Build history of the part. All positions in model axes, mm. A direction names the side the tool comes from. Round coordinates to 2 decimals unless told otherwise and drop trailing zeros. Write each loop counter-clockwise with the first axis right and the second up, starting at its lowest first coordinate (ties: lowest second). Pieces come first, ordered by that corner, then holes.
from build123d import *

# Parameters (mm, degrees)
SKETCH1_W                                      = 127
SKETCH1_H                                      = 12.7
BOSS_EXTRUDE1_DEPTH                            = 38.1
SKETCH3_R                                      = 4.445
CUT_EXTRUDE3_DEPTH                             = 2.54
CUT_EXTRUDE4_DEPTH                             = 13.208
CUT_EXTRUDE4_DEPTH_BACK                        = 13.208
SKETCH2_R                                      = 7.9756
SKETCH2_R_2                                    = 8.1026
SKETCH6_R                                      = 5.08
CUT_EXTRUDE5_DEPTH                             = 38.1
F_11_64_0_17188_DIAMETER_HOLE1_D               = 4.365752
F_11_64_0_17188_DIAMETER_HOLE1_DEPTH           = 25.4
F_11_64_0_17188_DIAMETER_HOLE1_TIP             = 1.311604225
F_11_64_0_17188_DIAMETER_HOLE1_ON_FACE_2_D     = 4.365752
F_11_64_0_17188_DIAMETER_HOLE1_ON_FACE_2_DEPTH = 25.4
F_11_64_0_17188_DIAMETER_HOLE1_ON_FACE_2_TIP   = 1.311604225


with BuildPart() as part:
    # Sketch1 → Boss-Extrude1 (new body)
    with BuildSketch(Plane(origin=(0, 0, 0), x_dir=(1, 0, 0), z_dir=(0, 1, 0))):
        with Locations((0, -6.35)):
            Rectangle(SKETCH1_W, SKETCH1_H)
    extrude(amount=BOSS_EXTRUDE1_DEPTH)

    # Sketch3 → Cut-Extrude3 (cut)
    with BuildSketch(Plane(origin=(0, 0, 0), x_dir=(-1, 0, 0), z_dir=(0, 0, -1))):
        with Locations((-58.039, 31.75)):
            Circle(SKETCH3_R)
        with Locations((-58.039, 6.35)):
            Circle(SKETCH3_R)
        with Locations((-31.009232106, 31.75)):
            Circle(SKETCH3_R)
        with Locations((-31.009232106, 6.35)):
            Circle(SKETCH3_R)
        with Locations((31.009232106, 31.75)):
            Circle(SKETCH3_R)
        with Locations((31.009232106, 6.35)):
            Circle(SKETCH3_R)
        with Locations((58.039, 31.75)):
            Circle(SKETCH3_R)
        with Locations((58.039, 6.35)):
            Circle(SKETCH3_R)
    extrude(amount=-CUT_EXTRUDE3_DEPTH, mode=Mode.SUBTRACT)

    # Sketch2 → Cut-Extrude4 (cut, two sides: drawn at the far end of the back side and taken through both)
    with BuildSketch(Plane(origin=(0, 19.05, 0), x_dir=(1, 0, 0), z_dir=(0, 1, 0)).offset(-CUT_EXTRUDE4_DEPTH_BACK)):
        with Locations((-44.45, -13.97)):
            Circle(SKETCH2_R)
        with Locations((44.45, -13.97)):
            Circle(SKETCH2_R_2)
    extrude(amount=CUT_EXTRUDE4_DEPTH + CUT_EXTRUDE4_DEPTH_BACK, mode=Mode.SUBTRACT)

    # Sketch6 → Cut-Extrude5 (cut)
    with BuildSketch(Plane(origin=(0, 38.1, 0), x_dir=(1, 0, 0), z_dir=(0, 1, 0))):
        with Locations((-44.45, -13.97)):
            Circle(SKETCH6_R)
        with Locations((44.45, -13.97)):
            Circle(SKETCH6_R)
    extrude(amount=-CUT_EXTRUDE5_DEPTH, mode=Mode.SUBTRACT)

    # 11/64 (0.17188) Diameter Hole1
    with Locations(Plane(origin=(58.039, 31.75, 0), x_dir=(-1, 0, 0), z_dir=(0, 0, -1))):
        with Locations((0, 0), (27.029767894, 0), (27.029767894, -25.4), (89.048232106, -25.4), (116.078, 0)):
            Hole(F_11_64_0_17188_DIAMETER_HOLE1_D / 2, depth=F_11_64_0_17188_DIAMETER_HOLE1_DEPTH)
            with Locations((0, 0, -(F_11_64_0_17188_DIAMETER_HOLE1_DEPTH + F_11_64_0_17188_DIAMETER_HOLE1_TIP / 2))):  # 118° drill point
                Cone(0, F_11_64_0_17188_DIAMETER_HOLE1_D / 2, F_11_64_0_17188_DIAMETER_HOLE1_TIP, mode=Mode.SUBTRACT)

    # 11/64 (0.17188) Diameter Hole1 on face 2
    with Locations(Plane(origin=(58.039, 6.35, 2.54), x_dir=(-1, 0, 0), z_dir=(0, 0, -1))):
        with Locations((0, 0), (89.048232106, 25.4), (116.078, 0)):
            Hole(F_11_64_0_17188_DIAMETER_HOLE1_ON_FACE_2_D / 2, depth=F_11_64_0_17188_DIAMETER_HOLE1_ON_FACE_2_DEPTH)
            with Locations((0, 0, -(F_11_64_0_17188_DIAMETER_HOLE1_ON_FACE_2_DEPTH + F_11_64_0_17188_DIAMETER_HOLE1_ON_FACE_2_TIP / 2))):  # 118° drill point
                Cone(0, F_11_64_0_17188_DIAMETER_HOLE1_ON_FACE_2_D / 2, F_11_64_0_17188_DIAMETER_HOLE1_ON_FACE_2_TIP, mode=Mode.SUBTRACT)


solid = part.part
1) Slice it at A-A (z = 3.75). Count the separate pieces of the cut face and the enclosed holes in it, plus the area to 3 significant figures.
Results:
separate pieces: 1
enclosed holes: 8
area: 4,720 mm2
2) Wall check: L1, parallel to Y at x = -58, z = 2.5; L2, parallel to X at y = 26, z = 7.75; L3, parallel to Y at x = 57, z = 1.5. Give the ranges that are in metal, low to high.
Results:
L1: y = 0 to 1.91, 10.79 to 27.31, 36.19 to 38.1
L2: x = -63.5 to -49.44, -39.46 to 39.26, 49.64 to 63.5
L3: y = 0 to 2.03, 10.67 to 27.43, 36.07 to 38.1
3) Slice it at B-B (y = 13). Write the cut outline in (x, z).
Results:
outline: (-63.5, 0) - (63.5, 0) - (63.5, 12.7) - (52.45, 12.7) arc R8.1 cw to (36.45, 12.7) - (-36.58, 12.7) arc R7.98 cw to (-52.32, 12.7) - (-63.5, 12.7) - close
4) Pin check, flat tip, straight feed: pin 1 Ø7 at (x, y) = (-58.039, 31.75) entering from -Z. Stop position of the tip, or through.
Results:
pin 1: stops at z = 2.54
5) Slice it at C-C (x = -47.5). Write the cut outline in (y, z), plus the area to 3 significant figures.
Results:
outline: (0, 0) - (38.1, 0) - (38.1, 9.91) - (32.26, 9.91) - (32.26, 6.6) - (5.84, 6.6) - (5.84, 9.91) - (0, 9.91) - close
area: 290 mm2
6) Mould opens along Y. For faces 1 (the cylindrical face through (-35.249, 33.085, 1.252)), 2 (the cylindrical face through (44.54, 2.96, 8.89)) say: released by +Y, released by -Y, zero draft, split by the parting line, or undercut.
Results:
face 1: undercut
face 2: zero draft
7) Which spindle directions (+Z, -Z, +X, -X, +Y, -Y) get a long thin tool onto all of the face, cutting with end or side? Do faces 3 (the cylindrical face through (-28.93, 7.01, 7.69)), 4 (the cylindrical face through (34.29, 9.35, 1.25)), 5 (the cylindrical face through (44.61, 18.87, 5.87)). Say none if no direction does.
Results:
face 3: +Z, -Z
face 4: -Z
face 5: +Z
